Input: dimensioned drawing with shaded views. Units: mm. Origin: part minimum x, y, z. A direction names the side the tool comes from. Round coordinates to 2 decimals unless told otherwise and drop trailing zeros. Order: outer loops, then holes, each group sorted by start corner. A loop starts at its lowest first (then second) coordinate and runs counter-clockwise, first axis right, second up. Notation, with made-up numbers: (84.25, 40.25) - (95.25, 40.25) arc R10 ccw to (95.25, 44.25) - close; hole circle Ø5 at (21, -10.75). An arc over 180 degrees is marked (long way). Put each result on its own line as item: value. Start each with the question number.
(1) Section A-A (z = 10.5). Output: boundary loops of the cut face in (x, y), and give its area (3 significant figures).
(2) Section D-D (y = 7.5). Output: boundary loops of the cut face in (x, z), and give its area (3 significant figures).
(3) Material intervals for L1, parallel to X at y = 6.25, z = 6.5; L2, parallel to X at y = 2.5, z = 6.5; L3, parallel to X at y = 6, z = 11, sorted ascending. Write a range as [from, to].
(4) Section B-B (x = 4). Output: boundary loops of the cut face in (y, z).
(5) Pull-direction query (X, two-part tool) for the marked faces 1 and 2; classes: released by +X, released by -X, zero draft, split by the parting line, or undercut.
(6) Pin query (flat end, axial travel): P1, Ø2.5, axis at y = 8.5, z = 9, coming from the -X side; P2, Ø6.5, axis at x = 41, z = 9, coming from the +Y side; P3, Ø2.5, axis at y = 6.5, z = 8, coming from the +X side. Return the tip coordinate at first contact, or that it passes through.
(7) Access query for the marked faces 3, 4 and 5. Directions: +Z, -Z, +X, -X, +Y, -Y. A direction counts if a zero-diameter tool reaches every point of the face in a straight line with its end or side. Return the directions, or none.
(8) Section C-C (y = 2.25). Output: boundary loops of the cut face in (x, z).
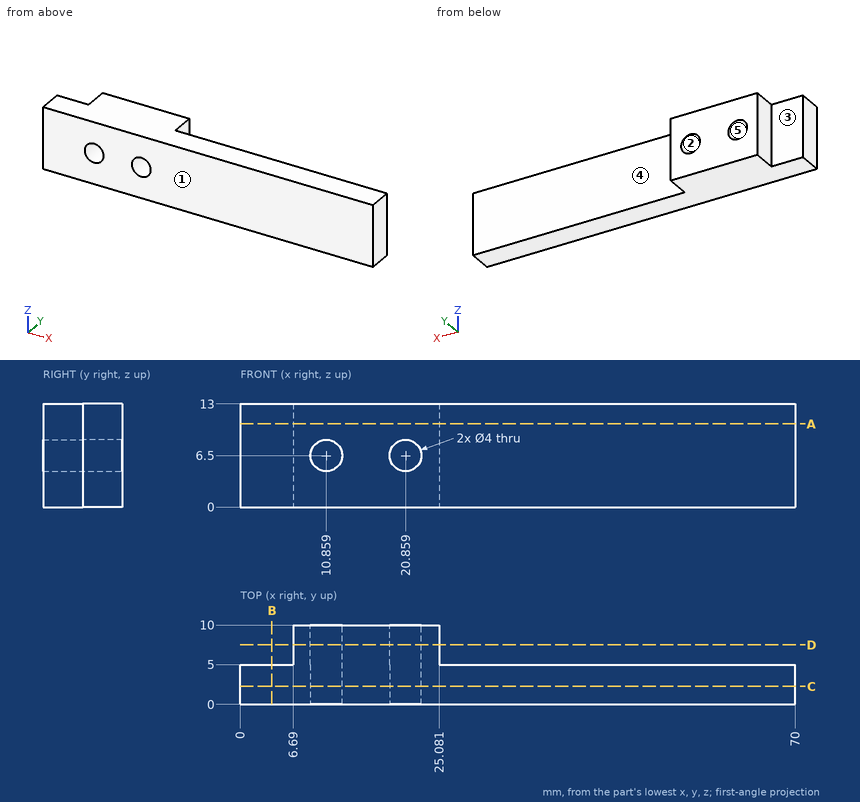
Checks:
1. outline: (0, 0) - (70, 0) - (70, 5) - (25.08, 5) - (25.08, 10) - (6.69, 10) - (6.69, 5) - (0, 5) - close
1. area: 442 mm²
2. outline: (6.69, 0) - (25.08, 0) - (25.08, 13) - (6.69, 13) - close; hole circle Ø4 at (10.86, 6.5); hole circle Ø4 at (20.86, 6.5)
2. area: 214 mm²
3. L1: x = [6.69, 8.86], [12.86, 18.86], [22.86, 25.08]
3. L2: x = [0, 8.86], [12.86, 18.86], [22.86, 70]
3. L3: x = [6.69, 25.08]
4. outline: (0, 0) - (5, 0) - (5, 13) - (0, 13) - close
5. face 1: zero draft
5. face 2: undercut
6. P1: stops at x = 6.69
6. P2: stops at y = 5
6. P3: stops at x = 25.08
7. face 3: +Z, -Z, -X, +Y
7. face 4: +Z, -Z, +X, +Y
7. face 5: +Y, -Y
8. outline: (0, 0) - (70, 0) - (70, 13) - (0, 13) - close; hole circle Ø4 at (10.86, 6.5); hole circle Ø4 at (20.86, 6.5)
